Geometry check sheet. Reference: the model listing, model coordinates, mm. A direction names the side the tool comes from. Round coordinates to 2 decimals unless told otherwise and drop trailing zeros. Order: outer loops, then holes, each group sorted by start corner. A loop starts at its lowest first (then second) coordinate and runs counter-clockwise, first axis right, second up. Notation, with made-up numbers: (74, 86.25) - (105, 86.25) arc R16 ccw to (105, 99.25) - close; hole circle Ø8 at (87.25, 45). An arc over 180 degrees is marked (long way). Return JSON: item names as keys, results as strings. Group by question number.
Q1. Gauge pin test, flat ends, axial feed: pin 1 Ø0.5 at (x, z) = (14, -0.5) entering from -Y; pin 2 Ø6 at (x, y) = (14, 14.5) entering from -Z; pin 3 Ø4 at (x, z) = (6, 0.5) entering from +Y; pin 4 Ø6 at (x, z) = (9, -3.5) entering from -Y. Record the tip position at first contact, or that the pin passes through.
Q2. Sectioned sample at C-C, the plane y = 25. Record the cut outline in (x, z).
Q3. Sectioned sample at B-B, the plane z = 2.25. Record the cut outline in (x, y) (3 decimals), then the cut area to 3 significant figures.
Q4. Sectioned sample at A-A, the plane x = 36.5. Record the cut outline in (y, z), then the cut area to 3 significant figures.
Q5. Material ranges on line 1 along Z through (x, y) = (40, 33); line 2 along Y through (x, z) = (43, -1.5); line 3 along Y through (x, z) = (21, 1), recorded low to high.
Q6. Sectioned sample at D-D, the plane y = -8. Record the cut outline in (x, z) (3 decimals).
Q7. Draft check along X on faces 4 (the flat face through (48, 32, 0)), 5 (the cylindrical face through (13.606, -5.423, 0.375)), 6 (the flat face through (7, 12, -5)), 7 (the cylindrical face through (-4.683, -3.751, -0.07)). Enter one of: pulls with the +X half, pulls with the -X half, needs draft (parallel to the pull), parting line crosses it, or undercut.
Q8. Tool access check on faces 1 (the flat face through (40.679, 34.493, -3.318)), 2 (the flat face through (21, -10.6, -1.2)), 3 (the cylindrical face through (18.983, -7.177, 0.375)). Record the directions out of +Z, -Z, +X, -X, +Y, -Y that give a thin tool (end or side, any length) a straight path to the whole face; none if there is none.
Autodesk Inventor part; units mm, degrees
ref_plane "YZ Plane" through (0, 0, 0) normal (1, 0, 0) x (0, 1, 0)
ref_plane "XZ Plane" through (0, 0, 0) normal (0, 1, 0) x (-1, 0, 0)
ref_plane "XY Plane" through (0, 0, 0) normal (0, 0, 1) x (1, 0, 0)
sketch "Sketch1" plane through (0, 0, 0) normal (0, 0, 1) x (1, 0, 0)
  line L0 (40, 15) -> (40, 0) construction
  circle A0 centre (-2.6718, 25) radius 1.55
  circle A1 centre (0, 0) radius 1.55
  arc A2 (2.1334, 28.593) -> (-3.4383, 30.9508) centre (-2.6718, 25) ccw construction
  arc A3 (-5.966, -0.6376) -> (-2.0133, -5.6521) centre (0, 0) ccw
  line L1 (-8.6378, 24.3624) -> (-5.966, -0.6376)
  line L2 (0, -6) -> (28, -6) construction
  line L3 (40, 0) -> (48, 0) construction
  line L4 (48, 0) -> (48, -6) construction
  line L5 (48, -6) -> (48, -11)
  line L6 (48, -11) -> (41.3764, -11)
  line L7 (13, -11) -> (-2.0133, -5.6521)
  line L8 (28, -6) -> (48, -6)
  line L9 (28, 30) -> (48, 30)
  line L10 (48, 30) -> (48, 35)
  line L11 (48, 35) -> (41.3764, 35)
  line L12 (48, -6) -> (48, 30) construction
  arc A4 (-8.6378, 24.3624) -> (2.1334, 28.593) centre (-2.6718, 25) ccw construction
  arc A5 (0, -6) -> (-5.966, -0.6376) centre (0, 0) ccw construction
  line L13 (28, -6) -> (28, 30) construction
  line L14 (28, 35) -> (-3.4383, 30.9508)
  arc A6 (-3.4383, 30.9508) -> (-8.6378, 24.3624) centre (-2.6718, 25) ccw
  line L15 (28, 35) -> (28, 30) construction
  arc A7 (28, 30) -> (28, -6) centre (28, 12) ccw
  line L16 (40, 15) -> (40, 35) construction
  line L17 (38.6236, 35) -> (40, 34)
  line L18 (40, 34) -> (41.3764, 35)
  line L19 (38.6236, 35) -> (41.3764, 35) construction
  line L20 (40, 34) -> (40, 35) construction
  line L21 (41.3764, -11) -> (40, -10)
  line L22 (40, -10) -> (38.6236, -11)
  line L23 (41.3764, -11) -> (38.6236, -11) construction
  line L24 (40, -10) -> (40, -11) construction
  line L25 (40, 0) -> (40, -11) construction
  line L26 (21.5514, -11) -> (20.175, -10)
  line L27 (20.175, -10) -> (18.7986, -11)
  line L28 (20.175, -10) -> (20.175, -11) construction
  line L29 (20.175, -10) -> (40, -10) construction
  line L30 (17.5514, -11) -> (16.175, -10)
  line L31 (16.175, -10) -> (14.7986, -11)
  line L32 (16.175, -10) -> (20.175, -10) construction
  line L33 (16.175, -10) -> (16.175, -11) construction
  line L34 (14.7986, -11) -> (13, -11)
  line L35 (17.5514, -11) -> (14.7986, -11) construction
  line L36 (21.5514, -11) -> (38.6236, -11)
  line L37 (17.5514, -11) -> (18.7986, -11)
  line L38 (18.7986, -11) -> (21.5514, -11) construction
  line L39 (38.6236, 35) -> (28, 35)
  line L40 (41.3764, 35) -> (38.6236, 35) construction
  arc A8 (-2.0133, -5.6521) -> (0, -6) centre (0, 0) ccw construction
  dimension "d0" = 3.1
  dimension "d1" = 12
  dimension "d4" = 5
  dimension "d6" = 15
  dimension "d7" = 36
  dimension "d40" = 108
  dimension "d41" = 1
  dimension "d42" = 108
  dimension "d43" = 1
  dimension "d46" = 108
  dimension "d48" = 19.825
  dimension "d49" = 108
  dimension "d51" = 4
  dimension "d52" = 12
  dimension "d53" = 8
extrude "Extrusion1" add sketch "Sketch1" along normal mid plane 10
ref_plane "Work Plane1" through (0, 0, 0) normal (0, 0, 1) x (1, 0, 0)
sketch "Sketch4" plane through (0, 0, 0) normal (0, 1, 0) x (-1, 0, 0)
  line L0 (-40, -5) -> (-40, 5)
  line L1 (-20.175, -5) -> (-20.175, 5)
  line L2 (-14.7986, -5) -> (-14.7986, 5)
  circle A0 centre (-40, 0) radius 1.5
  circle A1 centre (-20.175, 0) radius 1.25
  circle A2 centre (-14.7986, 0) radius 1.25
  point P0 (0, 0)
  dimension "d55" = 3
  dimension "d56" = 2.5
extrude "Extrusion4" cut sketch "Sketch4" against normal through all contours A1 L1 | L1 A1 | A2 L2 | L2 A2
extrude "Extrusion5" cut sketch "Sketch4" along normal through all both and the other way through all contours A0 L0 | L0 A0
chamfer "Chamfer1" [suppressed]
equation "\"d46\" = d42"
equation "\"d49\" = d50"
properties part number "bloco-dedo-1"
Reply:
{
 "1": {"pin 1": "y = 0", "pin 2": "through", "pin 3": "y = 32.42", "pin 4": "y = -10.64"},
 "2": {"outline": "(-8.67, -5) - (-4.22, -5) - (-4.22, 5) - (-8.67, 5) - close; (-1.12, -5) - (15.55, -5) - (15.55, 5) - (-1.12, 5) - close"},
 "3": {"outline": "(-8.638, 24.362) - (-5.966, -0.638) arc R6 ccw to (-2.013, -5.652) - (13, -11) - (14.799, -11) - (16.175, -10) - (17.551, -11) - (18.799, -11) - (20.175, -10) - (21.551, -11) - (38.624, -11) - (40, -10) - (41.376, -11) - (48, -11) - (48, -6) - (28, -6) arc R18 cw to (28, 30) - (48, 30) - (48, 35) - (41.376, 35) - (40, 34) - (38.624, 35) - (28, 35) - (-3.438, 30.951) arc R6 ccw to start; hole circle Ø3.1 at (-2.672, 25); hole circle Ø3.1 at (0, 0)", "area": "1,140 mm^2"},
 "4": {"outline": "(-11, -5) - (-6, -5) - (-6, 5) - (-11, 5) - close; (30, -5) - (35, -5) - (35, 5) - (30, 5) - close", "area": "100 mm^2"},
 "5": {"line 1": "-5 to -1.5, 1.5 to 5", "line 2": "-11 to -6, 30 to 35", "line 3": "-10.6 to -4.58, 28.58 to 34.1"},
 "6": {"outline": "(4.578, -5) - (48, -5) - (48, 5) - (4.578, 5) - close; hole circle Ø2.5 at (14.799, 0); hole circle Ø2.5 at (20.175, 0); hole circle Ø3 at (40, 0)"},
 "7": {"face 4": "pulls with the +X half", "face 5": "undercut", "face 6": "needs draft", "face 7": "pulls with the -X half"},
 "8": {"face 1": "+Z, -Z, +Y", "face 2": "+Z, -Z, -Y", "face 3": "-Y"}
}
